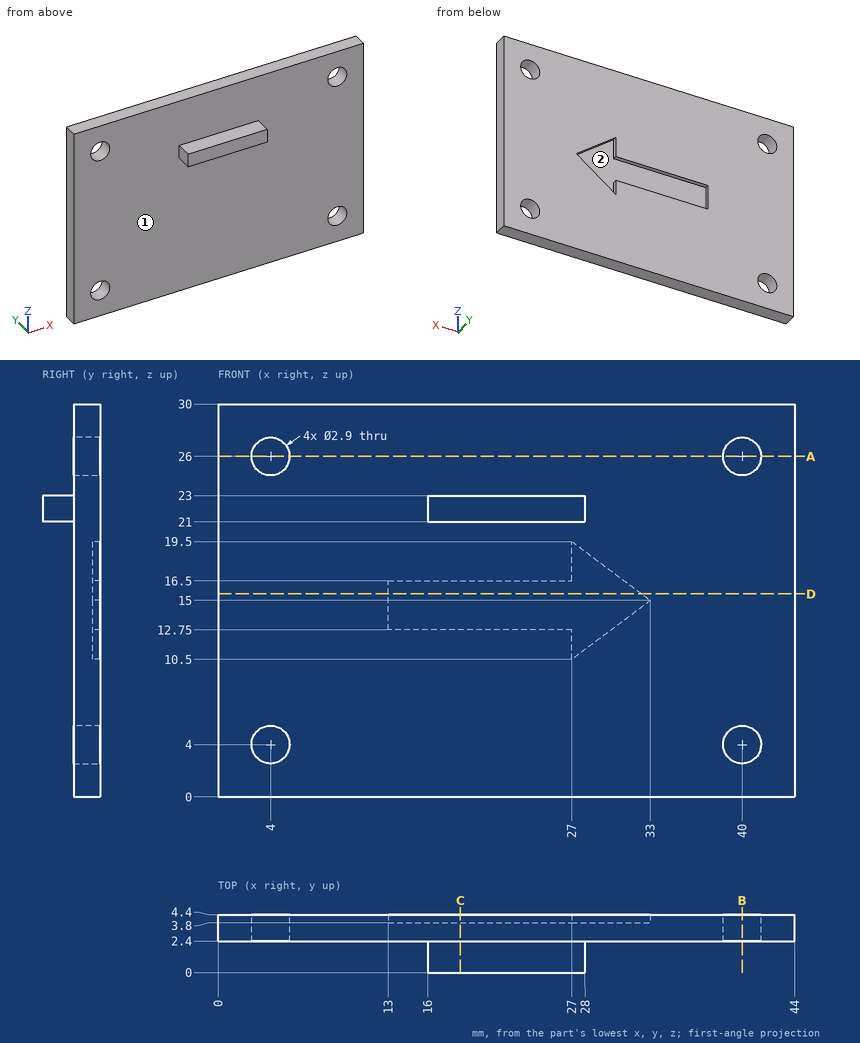
Check sheet for the drawn part. Datum: minimum x, y, z corner. Units: mm. Round coordinates to 2 decimals unless told otherwise and drop trailing zeros. Order: outer loops, then holes, each group sorted by start corner. A loop starts at its lowest first (then second) coordinate and runs counter-clockwise, first axis right, second up. Notation, with made-up numbers: (0.5, -13) -> (37.5, -13) arc R32 cw to (37.5, 13) -> close; hole circle Ø3 at (-2, 83). An arc over 180 degrees is marked (long way). Return JSON: item names as keys, results as strings. Group by question number.
Q1. Material ranges on probe 1 along Z at (x, y) = (40, 3.5); probe 2 along X at (y, z) = (3.85, 26); probe 3 along Z at (x, y) = (21, 4.05), recorded low to high. Write a range as from..to.
Q2. Section check B-B, the plane x = 40. Record the boundary of the cut face in (y, z), plus the area to 3 significant figures.
Q3. Section check C-C, the plane x = 18.5. Record the boundary of the cut face in (y, z), plus the area to 4 significant figures.
Q4. Gauge pin test, flat ends, axial feed: pin 1 (1.9 mm diameter, centred on x = 24, y = 0.5, fed in from +Z); pin 2 (6 mm diameter, centred on x = 12.5, z = 7.5, fed in from -Y); pin 3 (1 mm diameter, centred on x = 16.5, y = 1.5, fed in from -Z); pin 4 (2.5 mm diameter, centred on x = 40, z = 26, fed in from -Y). Record the tip position at first contact, or that the pin passes through.
Q5. Release check for a two-part mould opening along X. For the marked faces 1 and 2 record: released by +X, released by -X, zero draft, split by the parting line, or undercut.
Q6. Section check D-D, the plane z = 15.5. Record the boundary of the cut face in (x, y).
Q7. Section check A-A, the plane z = 26. Record the boundary of the cut face in (x, y), plus the area to 3 significant figures.
Numbers:
{
 "1": {"probe 1": "0..2.55, 5.45..24.55, 27.45..30", "probe 2": "0..2.55, 5.45..38.55, 41.45..44", "probe 3": "0..12.75, 16.5..30"},
 "2": {"outline": "(2.4, 0) -> (4.4, 0) -> (4.4, 2.55) -> (2.4, 2.55) -> close; (2.4, 5.45) -> (4.4, 5.45) -> (4.4, 24.55) -> (2.4, 24.55) -> close; (2.4, 27.45) -> (4.4, 27.45) -> (4.4, 30) -> (2.4, 30) -> close", "area": "48.4 mm^2"},
 "3": {"outline": "(0, 21) -> (2.4, 21) -> (2.4, 0) -> (4.4, 0) -> (4.4, 12.75) -> (3.8, 12.75) -> (3.8, 16.5) -> (4.4, 16.5) -> (4.4, 30) -> (2.4, 30) -> (2.4, 23) -> (0, 23) -> close", "area": "62.55 mm^2"},
 "4": {"pin 1": "z = 23", "pin 2": "y = 2.4", "pin 3": "z = 21", "pin 4": "through"},
 "5": {"face 1": "zero draft", "face 2": "undercut"},
 "6": {"outline": "(0, 2.4) -> (44, 2.4) -> (44, 4.4) -> (32.33, 4.4) -> (32.33, 3.8) -> (13, 3.8) -> (13, 4.4) -> (0, 4.4) -> close"},
 "7": {"outline": "(0, 2.4) -> (2.55, 2.4) -> (2.55, 4.4) -> (0, 4.4) -> close; (5.45, 2.4) -> (38.55, 2.4) -> (38.55, 4.4) -> (5.45, 4.4) -> close; (41.45, 2.4) -> (44, 2.4) -> (44, 4.4) -> (41.45, 4.4) -> close", "area": "76.4 mm^2"}
}
